The listing builds one solid part. Answer for the finished solid, in the listing's coordinates (mm). A direction names the side the tool comes from. Coordinates: 2 decimals unless noted, no trailing zeros. Order: outer loops, then holes, each group sorted by start corner. A loop starts at its lowest first (then second) coordinate and runs counter-clockwise, first axis right, second up. Notation, with made-up numbers: (50.5, -10) -> (74.5, -10) arc R18 ccw to (74.5, -1) -> close; hole circle Ø11 at (64, 43). An arc over 180 degrees is marked (long way). Answer in a Markdown table with one row per item.
```python
from build123d import *

# Parameters (mm, degrees)
SKETCH1_R                                       = 2
BOSS_EXTRUDE1_DEPTH                             = 20
CSK_FOR_M5_FLAT_HEAD_MACHINE_SCREW1_D           = 5.5
CSK_FOR_M5_FLAT_HEAD_MACHINE_SCREW1_CSINK_D     = 10.4
CSK_FOR_M5_FLAT_HEAD_MACHINE_SCREW1_CSINK_ANGLE = 90
BOSS_EXTRUDE2_DEPTH                             = 10
FILLET3_R                                       = 8


with BuildPart() as part:
    # Sketch1 → Boss-Extrude1 (new body)
    with BuildSketch(Plane.XY):
        with BuildLine():
            Line((0, -9.75), (-11.25, -9.75))
            ThreePointArc((-11.25, -9.75), (-13.371320344, -8.871320344), (-14.25, -6.75))
            Line((-14.25, -6.75), (-14.25, 6.75))
            ThreePointArc((-14.25, 6.75), (-13.371320344, 8.871320344), (-11.25, 9.75))
            Line((-11.25, 9.75), (0, 9.75))
            Line((0, 9.75), (0, 12))
            Line((0, 12), (-11.25, 12))
            ThreePointArc((-11.25, 12), (-13.080137287, 11.670680594), (-14.680674679, 10.724037147))
            Line((-14.680674679, 10.724037147), (-23.346538156, 3.243040543))
            ThreePointArc((-23.346538156, 3.243040543), (-23.651402422, 3.062727506), (-24, 3))
            Line((-24, 3), (-36, 3))
            Line((-36, 3), (-36, -10.5))
            Line((-36, -10.5), (0, -10.5))
            Line((0, -10.5), (0, -9.75))
        make_face()
        with Locations((-20, 0)):
            Circle(SKETCH1_R, mode=Mode.SUBTRACT)
    extrude(amount=BOSS_EXTRUDE1_DEPTH)

    # CSK for M5 Flat Head Machine Screw1 (through all)
    with Locations(Plane(origin=(0, 3, 0), x_dir=(1, 0, 0), z_dir=(0, 1, 0))):
        with Locations((-30, -10)):
            CounterSinkHole(CSK_FOR_M5_FLAT_HEAD_MACHINE_SCREW1_D / 2, CSK_FOR_M5_FLAT_HEAD_MACHINE_SCREW1_CSINK_D / 2, counter_sink_angle=CSK_FOR_M5_FLAT_HEAD_MACHINE_SCREW1_CSINK_ANGLE)

    # Sketch7 → Boss-Extrude2 (add)
    with BuildSketch(Plane.XY.offset(20)):
        with BuildLine():
            Line((0, 9.75), (0, 12))
            Line((0, 12), (-11.25, 12))
            ThreePointArc((-11.25, 12), (-13.080137287, 11.670680594), (-14.680674679, 10.724037147))
            ThreePointArc((-14.680674679, 10.724037147), (-16.023549102, 8.93534413), (-16.5, 6.75))
            Line((-16.5, 6.75), (-16.5, -10.5))
            Line((-16.5, -10.5), (0, -10.5))
            Line((0, -10.5), (0, -9.75))
            Line((0, -9.75), (-11.25, -9.75))
            ThreePointArc((-11.25, -9.75), (-13.371320344, -8.871320344), (-14.25, -6.75))
            Line((-14.25, -6.75), (-14.25, 6.75))
            ThreePointArc((-14.25, 6.75), (-13.371320344, 8.871320344), (-11.25, 9.75))
            Line((-11.25, 9.75), (0, 9.75))
        make_face()
    extrude(amount=BOSS_EXTRUDE2_DEPTH)

    # Fillet3
    fillet3_edges = [part.edges().sort_by_distance(p)[0] for p in [
        (-36, -3.75, 0),
        (-36, -3.75, 20),
    ]]
    fillet(fillet3_edges, radius=FILLET3_R)

    # Mirror1: part across plane


with BuildPart() as part_1:
    add(part.part)
    add(part.part.mirror(Plane(origin=(0, 0, 0), x_dir=(0, 0, 1), z_dir=(1, 0, 0))))


solid = part_1.part
```
(1) Which of the six approach directions +Z, -Z, +X, -X, +Y, -Y give full straight-line access (tool end or side, diameter ignored) to faces 1 (the flat face through (0, 12, 15)), 2 (the flat face through (14.25, 0, 15)), 3 (the flat face through (-24.6, 3, 9.9))?
Check values:
| item | result |
|---|---|
| face 1 | +Z, -Z, +X, -X, +Y |
| face 2 | +Z, -Z |
| face 3 | +Z, -Z, -X, +Y |
(2) A cutting plane is placed at B-B, the plane y = -0.75. Determine the outline of the cut face in (x, z).
Check values:
| item | result |
|---|---|
| outline | (-36, 8) arc R8 ccw to (-28, 0) -> (-21.85, 0) -> (-21.85, 20) -> (-28, 20) arc R8 ccw to (-36, 12) -> close; (-18.15, 0) -> (-14.25, 0) -> (-14.25, 30) -> (-16.5, 30) -> (-16.5, 20) -> (-18.15, 20) -> close; (14.25, 0) -> (18.15, 0) -> (18.15, 20) -> (16.5, 20) -> (16.5, 30) -> (14.25, 30) -> close; (21.85, 0) -> (28, 0) arc R8 ccw to (36, 8) -> (36, 12) arc R8 ccw to (28, 20) -> (21.85, 20) -> close; hole circle Ø5.5 at (-30, 10); hole circle Ø5.5 at (30, 10) |
(3) A cutting plane is placed at A-A, the plane z = 10. Count the separate pieces of the cut face and the enclosed holes in it, then the cut area to 3 significant figures.
Check values:
| item | result |
|---|---|
| separate pieces | 3 |
| enclosed holes | 3 |
| area | 569 mm² |
(4) A cutting plane is placed at D-D, the plane y = 7.75. Determine the outline of the cut face in (x, z), then the cut area to 3 significant figures.
Check values:
| item | result |
|---|---|
| outline | (-18.13, 0) -> (-14.08, 0) -> (-14.08, 30) -> (-16.4, 30) -> (-16.4, 20) -> (-18.13, 20) -> close; (14.08, 0) -> (18.13, 0) -> (18.13, 20) -> (16.4, 20) -> (16.4, 30) -> (14.08, 30) -> close |
| area | 208 mm² |
(5) A cutting plane is placed at C-C, the plane x = 20. Determine the outline of the cut face in (y, z), then the cut area to 3 significant figures.
Check values:
| item | result |
|---|---|
| outline | (-10.5, 0) -> (-2, 0) -> (-2, 20) -> (-10.5, 20) -> close; (2, 0) -> (6.13, 0) -> (6.13, 20) -> (2, 20) -> close |
| area | 253 mm² |
(6) For a pull along Z with two mould halves and no side action, classify faces 4 (the flat face through (-21, -2, 20)), 5 (the conical face through (32.65, 0.67, 11.1)), 6 (the cylindrical face through (-27.253, -5.052, 9.879)), 7 (the flat face through (18.95, 7.04, 9.86)) as released by +Z, released by -Z, zero draft, split by the parting line, or undercut.
Check values:
| item | result |
|---|---|
| face 4 | released by +Z |
| face 5 | undercut |
| face 6 | undercut |
| face 7 | zero draft |
(7) Flat-ended cylindrical pins translate along their axes: pin 1 (5 mm diameter, centred on y = -3.5, z = 24, fed in from +X); pin 2 (12 mm diameter, centred on x = 18, z = 20, fed in from +Y); pin 3 (6 mm diameter, centred on x = 6.5, y = 7, fed in from -Z); pin 4 (7 mm diameter, centred on y = 2.5, z = 19, fed in from +X). Find the tip coordinate at first contact, or state that the pin passes through.
Check values:
| item | result |
|---|---|
| pin 1 | x = 16.5 |
| pin 2 | y = 11.95 |
| pin 3 | z = 0 |
| pin 4 | x = 35.19 |
(8) Find the intervals of material crossed by line 1 along X through (y, z) = (-6, 10); line 2 along X through (y, z) = (3.25, 20.25); line 3 along Y through (x, z) = (-1, 5.5), in increasing order. Write a range as from..to.
Check values:
| item | result |
|---|---|
| line 1 | -36..-32.75, -27.25..-14.25, 14.25..27.25, 32.75..36 |
| line 2 | -16.5..-14.25, 14.25..16.5 |
| line 3 | -10.5..-9.75, 9.75..12 |
